Could you check a few things on this model? Use its own coordinates, in mm. Coordinates: 2 decimals unless noted, no trailing zeros. Write each loop counter-clockwise with the first axis right and the second up, starting at its lowest first coordinate (ties: lowest second). Pieces come first, ordered by that corner, then holes. Notation, with made-up numbers: M 21.5,12.5 L 35.5,12.5 A14 ccw 35.5,17.5 Z; hole C 11,57 d10. An arc over 180 degrees is marked long. Write item = value, one per line.
```python
from build123d import *

# Parameters (mm, degrees)
SKETCH_1_R          = 2
EXTRUDE_1_DEPTH     = 20
SKETCH_2_W          = 18
SKETCH_2_H          = 18
CUT_EXTRUDE_1_DEPTH = 259.043348145


with BuildPart() as part:
    # 草图1 → 凸台-拉伸1 (new body)
    with BuildSketch(Plane(origin=(0, 0, 0), x_dir=(1, 0, 0), z_dir=(0, 1, 0))):
        Polygon((-10.212466243, 128.533123378), (9.787533757, 128.533123378), (9.787533757, -116.984211541), (-10.212466243, -128.531216924), align=None)
        with Locations(Location((-0.212466243, -111.466876622, 0), (0, 0, 270))):
            Circle(SKETCH_1_R, mode=Mode.SUBTRACT)
        with Locations(Location((-0.212466243, -101.466876622, 0), (0, 0, 270))):
            Circle(SKETCH_1_R, mode=Mode.SUBTRACT)
        with Locations(Location((-0.212466243, 107.533123378, 0), (0, 0, 270))):
            Circle(SKETCH_1_R, mode=Mode.SUBTRACT)
        with Locations(Location((-0.212466243, 119.533123378, 0), (0, 0, 270))):
            Circle(SKETCH_1_R, mode=Mode.SUBTRACT)
    extrude(amount=EXTRUDE_1_DEPTH)

    # 草图2 → 切除-拉伸1 (cut, through all)
    with BuildSketch(Plane(origin=(0, 0, -128.533123378), x_dir=(-1, 0, 0), z_dir=(0, 0, -1))):
        with Locations((0, 10)):
            Rectangle(SKETCH_2_W, SKETCH_2_H)
    extrude(amount=-CUT_EXTRUDE_1_DEPTH, mode=Mode.SUBTRACT)


solid = part.part
```
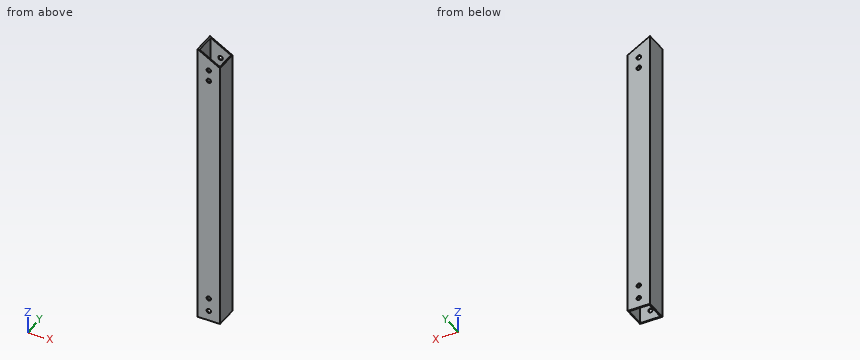
Item 1: I'm going to push a flat-ended pin straight in: P1, Ø3.5, axis at x = -0.21, z = -107.53, coming from the +Y side. Where does the tip first touch, or does it pass through?
Numbers:
P1 = through
Item 2: Imagine slicing it at B-B (z = -87). Write out the boundary of the cut face in (x, y), and give its area (3 significant figures).
Numbers:
outline = M -10.21,0 L 9.79,0 L 9.79,20 L -10.21,20 Z; hole M -9,1 L 9,1 L 9,19 L -9,19 Z
area = 76.0 mm²
Item 3: Imagine slicing it at A-A (y = 10). Write out the boundary of the cut face in (x, z), and give its area (3 significant figures).
Numbers:
outline = M -10.21,-128.53 L -9,-128.53 L -9,127.83 L -10.21,128.53 Z; M 9,-128.53 L 9.79,-128.53 L 9.79,116.98 L 9,117.44 Z
area = 505 mm²
Item 4: If I drill on line 1 along Y through (x, z) = (6.75, 3); line 2 along X through (y, z) = (9, -107.5), over which ranges is the centre line in solid material (lowest first)?
Numbers:
line_1 = 0 to 1, 19 to 20
line_2 = -10.21 to -9, 9 to 9.79
Item 5: Imagine slicing it at C-C (x = -6). Write out the boundary of the cut face in (y, z).
Numbers:
outline = M 0,-128.53 L 1,-128.53 L 1,126.1 L 0,126.1 Z; M 19,-128.53 L 20,-128.53 L 20,126.1 L 19,126.1 Z
